from build123d import *

# Parameters (mm, degrees)
SKETCH1_R           = 7
SKETCH1_R_2         = 4
BOSS_EXTRUDE1_DEPTH = 6
SKETCH2_R           = 7
BOSS_EXTRUDE2_DEPTH = 10
CUT_EXTRUDE1_DEPTH  = 8
SKETCH4_W           = 4.3
SKETCH4_H           = 6.3
CUT_EXTRUDE2_DEPTH  = 6
SKETCH5_OUTSIDE_W   = 21.092
SKETCH5_OUTSIDE_H   = 21.092
CUT_EXTRUDE3_DEPTH  = 8
BOSS_EXTRUDE3_DEPTH = 8
SKETCH9_R           = 7
CUT_EXTRUDE6_DEPTH  = 8
SKETCH10_W          = 9
SKETCH10_H          = 7
BOSS_EXTRUDE5_DEPTH = 9
SKETCH11_W          = 4.3
SKETCH11_H          = 6.3
CUT_EXTRUDE7_DEPTH  = 6
BOSS_EXTRUDE6_DEPTH = 8
SKETCH14_W          = 7
SKETCH14_H          = 9
BOSS_EXTRUDE7_DEPTH = 2.6
SKETCH15_W          = 4
SKETCH15_H          = 5
CUT_EXTRUDE10_DEPTH = 9
SKETCH16_R          = 1.5
CUT_EXTRUDE11_DEPTH = 6.6


with BuildPart() as part:
    # Sketch1 → Boss-Extrude1 (new body)
    with BuildSketch(Plane(origin=(0, 0, 0), x_dir=(1, 0, 0), z_dir=(0, 1, 0))):
        with Locations(Location((0, 0, 0), (0, 0, 270))):  # turned: the seam where the file's is
            Circle(SKETCH1_R)
        with Locations(Location((0, 0, 0), (0, 0, 270))):  # turned: the seam where the file's is
            Circle(SKETCH1_R_2, mode=Mode.SUBTRACT)
    extrude(amount=BOSS_EXTRUDE1_DEPTH)

    # Sketch2 → Boss-Extrude2 (add)
    with BuildSketch(Plane(origin=(0, 6, 0), x_dir=(1, 0, 0), z_dir=(0, 1, 0))):
        with Locations(Location((0, 0, 0), (0, 0, 270))):  # turned: the seam where the file's is
            Circle(SKETCH2_R)
    extrude(amount=BOSS_EXTRUDE2_DEPTH)

    # Sketch3 → Cut-Extrude1 (cut)
    with BuildSketch(Plane(origin=(0, 16, 0), x_dir=(1, 0, 0), z_dir=(0, 1, 0))):
        with BuildLine():
            Line((0, 7), (0, -7))
            ThreePointArc((0, -7), (-7, 0), (0, 7))
        make_face()
    extrude(amount=-CUT_EXTRUDE1_DEPTH, mode=Mode.SUBTRACT)

    # Sketch4 → Cut-Extrude2 (cut)
    with BuildSketch(Plane.ZY):
        with Locations((0, 12.15)):
            Rectangle(SKETCH4_W, SKETCH4_H)
    extrude(amount=-CUT_EXTRUDE2_DEPTH, mode=Mode.SUBTRACT)

    # Sketch5 outside → Cut-Extrude3 (cut)
    with BuildSketch(Plane(origin=(0, 16, 0), x_dir=(1, 0, 0), z_dir=(0, 1, 0))):
        Rectangle(SKETCH5_OUTSIDE_W, SKETCH5_OUTSIDE_H)
        with BuildLine():
            Line((0, 4), (5.744562647, 4))
            ThreePointArc((5.744562647, 4), (7, 0), (5.744562647, -4))
            Line((5.744562647, -4), (0, -4))
            Line((0, -4), (0, 4))
        make_face(mode=Mode.SUBTRACT)
    extrude(amount=-CUT_EXTRUDE3_DEPTH, mode=Mode.SUBTRACT)

    # Sketch7 → Boss-Extrude3 (add)
    with BuildSketch(Plane(origin=(0, 8, 0), x_dir=(1, 0, 0), z_dir=(0, 1, 0))):
        with BuildLine():
            Line((2, 6.708203932), (2, 11.708203932))
            Line((2, 11.708203932), (-2, 11.708203932))
            Line((-2, 11.708203932), (-2, 6.708203932))
            ThreePointArc((-2, 6.708203932), (0, 7), (2, 6.708203932))
        make_face()
        with BuildLine():
            Line((2, -6.708203932), (2, -11.708203932))
            Line((2, -11.708203932), (-2, -11.708203932))
            Line((-2, -11.708203932), (-2, -6.708203932))
            ThreePointArc((-2, -6.708203932), (0, -7), (2, -6.708203932))
        make_face()
    extrude(amount=-BOSS_EXTRUDE3_DEPTH)

    # Sketch9 → Cut-Extrude6 (cut)
    with BuildSketch(Plane(origin=(0, 16, 0), x_dir=(1, 0, 0), z_dir=(0, 1, 0))):
        Circle(SKETCH9_R)
    extrude(amount=-CUT_EXTRUDE6_DEPTH, mode=Mode.SUBTRACT)

    # Sketch10 → Boss-Extrude5 (add)
    with BuildSketch(Plane(origin=(0, 8, 0), x_dir=(1, 0, 0), z_dir=(0, 1, 0))):
        Rectangle(SKETCH10_W, SKETCH10_H)
    extrude(amount=BOSS_EXTRUDE5_DEPTH)

    # Sketch11 → Cut-Extrude7 (cut)
    with BuildSketch(Plane.ZY.offset(4.5)):
        with Locations((0, 12.5)):
            Rectangle(SKETCH11_W, SKETCH11_H)
    extrude(amount=-CUT_EXTRUDE7_DEPTH, mode=Mode.SUBTRACT)

    # Sketch13 → Boss-Extrude6 (add)
    with BuildSketch(Plane(origin=(0, 8, 0), x_dir=(1, 0, 0), z_dir=(0, 1, 0))):
        with BuildLine():
            Line((2, -6.708203932), (7.1, -6.708203932))
            Line((7.1, -6.708203932), (7.1, 6.708203932))
            Line((7.1, 6.708203932), (2, 6.708203932))
            ThreePointArc((2, 6.708203932), (7, 0), (2, -6.708203932))
        make_face()
    extrude(amount=-BOSS_EXTRUDE6_DEPTH)

    # Sketch14 → Boss-Extrude7 (add)
    with BuildSketch(Plane(origin=(4.5, 0, 0), x_dir=(0, 0, -1), z_dir=(1, 0, 0))):
        with Locations((0, 12.5)):
            Rectangle(SKETCH14_W, SKETCH14_H)
    extrude(amount=BOSS_EXTRUDE7_DEPTH)

    # Sketch15 → Cut-Extrude10 (cut, through all)
    with BuildSketch(Plane(origin=(0, 8, 0), x_dir=(1, 0, 0), z_dir=(0, 1, 0))):
        with Locations((0, 9.208203932)):
            Rectangle(SKETCH15_W, SKETCH15_H)
        with Locations((0, -9.208203932)):
            Rectangle(SKETCH15_W, SKETCH15_H)
    extrude(amount=-CUT_EXTRUDE10_DEPTH, mode=Mode.SUBTRACT)

    # Sketch16 → Cut-Extrude11 (cut, through all)
    with BuildSketch(Plane.ZY.offset(-1.5)):
        with Locations((0, 12.5)):
            Circle(SKETCH16_R)
    extrude(amount=-CUT_EXTRUDE11_DEPTH, mode=Mode.SUBTRACT)


solid = part.part
Input: part model. Units: mm. Frame: model coordinates. A direction names the side the tool comes from. Coordinates: 2 decimals unless noted, no trailing zeros. Loops run counter-clockwise (first coordinate to the right, second up) from the corner with the lowest first, then second, coordinate; pieces in that order, holes last.
(1) Section A-A on y = 12.5. Return the cut outline in (x, z).
(2) Section C-C on x = 0. Return the cut outline in (y, z).
(3) Section B-B on z = 0. Return the cut outline in (x, y).
(4) First-contact query: pin 1 Ø1.8 at (x, y) = (-3, 13) entering from +Z; pin 2 Ø5 at (x, z) = (0, 0) entering from -Y; pin 3 Ø3.5 at (y, z) = (11, 1) entering from -X. Flat tips, straight axial feed; report the tip coordinate or a pass-through.
(5) Section D-D on y = 3.25. Return the cut outline in (x, z).
(6) Pull-direction query (Y, two-part tool) for faces 1 (the face through (1, 17, 0)), 2 (the face through (2, 4, 6.708)), 3 (the face through (-2, 15.65, 0)); classes: released by +Y, released by -Y, zero draft, split by the parting line, or undercut.
(7) Set-up query: faces 4 (the face through (-2, 12, 2.15)), 5 (the face through (-4.5, 12.4, 2.4)), 6 (the face through (1, 12, 3.5)), 7 (the face through (0, 6, 0)), 8 (the face through (1, 12, -3.5)). Return all of +Z, -Z, +X, -X, +Y, -Y with unobstructed straight access to the full face (end or side cutting, diameter ignored); none if empty.
(8) Material intervals for probe 1 along Y at (x, z) = (4.05, 0); probe 2 along Z at (x, y) = (-0.5, 13.5); probe 3 along Y at (x, z) = (0, -2), sorted ascending.
Data:
1. outline: (-4.5, -3.5) - (7.1, -3.5) - (7.1, -1.5) - (1.5, -1.5) - (1.5, -2.15) - (-4.5, -2.15) - close; (-4.5, 2.15) - (1.5, 2.15) - (1.5, 1.5) - (7.1, 1.5) - (7.1, 3.5) - (-4.5, 3.5) - close
2. outline: (0, -6.71) - (8, -6.71) - (8, -3.5) - (17, -3.5) - (17, 3.5) - (8, 3.5) - (8, 6.71) - (0, 6.71) - (0, 4) - (6, 4) - (6, -4) - (0, -4) - close; hole (9.35, -2.15) - (15.65, -2.15) - (15.65, 2.15) - (9.35, 2.15) - close
3. outline: (-7, 0) - (-4, 0) - (-4, 6) - (4, 6) - (4, 0) - (7.1, 0) - (7.1, 11) - (1.5, 11) - (1.5, 9.35) - (-4.5, 9.35) - (-4.5, 8) - (-7, 8) - close; (-4.5, 15.65) - (1.5, 15.65) - (1.5, 14) - (7.1, 14) - (7.1, 17) - (-4.5, 17) - close
4. pin 1: stops at z = 3.5
4. pin 2: stops at y = 6
4. pin 3: stops at x = -4.5
5. outline: (-2, -6.71) - (7.1, -6.71) - (7.1, 6.71) - (-2, 6.71) arc R7 ccw to start; hole circle Ø8 at (0, 0)
6. face 1: released by +Y
6. face 2: zero draft
6. face 3: undercut
7. face 4: -X
7. face 5: +Z, -Z, -X, +Y
7. face 6: +Z, +X, -X, +Y
7. face 7: -Y
7. face 8: -Z, +X, -X, +Y
8. probe 1: y = 0 to 11, 14 to 17
8. probe 2: z = -3.5 to -2.15, 2.15 to 3.5
8. probe 3: y = 6 to 9.35, 15.65 to 17
